from build123d import *

# Parameters (mm, degrees)
SKETCH_1_R                = 4
EXTRUDE_1_DEPTH           = 5
EXTRUDE_2_DEPTH           = 12
EXTRUDE_2_DEPTH_BACK      = 12
EXTRUDE_3_DEPTH           = 16
EXTRUDE_3_DEPTH_BACK      = 16
SKETCH_2_3_R              = 4
CUT_EXTRUDE_1_DEPTH       = 9
CUT_EXTRUDE_1_DEPTH_BACK  = 9
SKETCH_2_4_R              = 4
SKETCH_2_5_R              = 25
EXTRUDE_4_DEPTH           = 9
EXTRUDE_4_TAPER           = 30
EXTRUDE_4_OTHER_WAY_DEPTH = 9
EXTRUDE_4_OTHER_WAY_TAPER = 30


with BuildPart() as part:
    # Sketch 1 → Extrude 1 (new body)
    with BuildSketch(Plane.XY):
        with BuildLine():
            Line((21.5, -35), (-21.5, -35))
            ThreePointArc((-21.5, -35), (-24.328427125, -33.828427125), (-25.5, -31))
            Line((-25.5, -31), (-25.5, 31))
            ThreePointArc((-25.5, 31), (-24.328427125, 33.828427125), (-21.5, 35))
            Line((-21.5, 35), (21.5, 35))
            ThreePointArc((21.5, 35), (24.328427125, 33.828427125), (25.5, 31))
            Line((25.5, 31), (25.5, -31))
            ThreePointArc((25.5, -31), (24.328427125, -33.828427125), (21.5, -35))
        make_face()
        with Locations((-17.5, 26.5)):
            Circle(SKETCH_1_R, mode=Mode.SUBTRACT)
        with Locations((17.5, 26.5)):
            Circle(SKETCH_1_R, mode=Mode.SUBTRACT)
        with Locations((17.5, -26.5)):
            Circle(SKETCH_1_R, mode=Mode.SUBTRACT)
        with Locations((-17.5, -26.5)):
            Circle(SKETCH_1_R, mode=Mode.SUBTRACT)
    extrude(amount=EXTRUDE_1_DEPTH)

    # Sketch 2 → Extrude 2 (add, two sides: drawn at the far end of the back side and taken through both)
    with BuildSketch(Plane(origin=(0, 0, 0), x_dir=(0, 0, -1), z_dir=(1, 0, 0)).offset(-EXTRUDE_2_DEPTH_BACK)):
        with BuildLine():
            ThreePointArc((23.824417981, -16.040481733), (18, 0), (23.824417981, 16.040481733))
            Line((23.824417981, 16.040481733), (0, 31))
            Line((0, 31), (0, -31))
            Line((0, -31), (23.824417981, -16.040481733))
        make_face()
        with BuildLine():
            ThreePointArc((43, -4), (39, 0), (43, 4))
            Line((43, 4), (23.824417981, 16.040481733))
            ThreePointArc((23.824417981, 16.040481733), (18, 0), (23.824417981, -16.040481733))
            Line((23.824417981, -16.040481733), (43, -4))
        make_face()
    extrude(amount=EXTRUDE_2_DEPTH + EXTRUDE_2_DEPTH_BACK)

    # Sketch 2_3 → Extrude 3 (add, two sides: drawn at the far end of the back side and taken through both)
    with BuildSketch(Plane(origin=(0, 0, 0), x_dir=(0, 0, -1), z_dir=(1, 0, 0)).offset(-EXTRUDE_3_DEPTH_BACK)):
        with Locations((43, 0)):
            Circle(SKETCH_2_3_R)
    extrude(amount=EXTRUDE_3_DEPTH + EXTRUDE_3_DEPTH_BACK)

    # Sketch 2_4 → Cut-Extrude 1 (cut, two sides: drawn at the far end of the back side and taken through both)
    with BuildSketch(Plane(origin=(0, 0, 0), x_dir=(0, 0, -1), z_dir=(1, 0, 0)).offset(-CUT_EXTRUDE_1_DEPTH_BACK)):
        with BuildLine():
            ThreePointArc((23.824417981, -16.040481733), (18, 0), (23.824417981, 16.040481733))
            Line((23.824417981, 16.040481733), (0, 31))
            Line((0, 31), (0, -31))
            Line((0, -31), (23.824417981, -16.040481733))
        make_face()
        with BuildLine():
            ThreePointArc((43, -4), (39, 0), (43, 4))
            Line((43, 4), (23.824417981, 16.040481733))
            ThreePointArc((23.824417981, 16.040481733), (18, 0), (23.824417981, -16.040481733))
            Line((23.824417981, -16.040481733), (43, -4))
        make_face()
        with BuildLine():
            Line((23.824417981, 16.040481733), (43, 4))
            ThreePointArc((43, 4), (45.828427125, 2.828427125), (47, 0))
            ThreePointArc((47, 0), (45.828427125, -2.828427125), (43, -4))
            Line((43, -4), (23.824417981, -16.040481733))
            ThreePointArc((23.824417981, -16.040481733), (51.532597773, -23.498824976), (68, 0))
            ThreePointArc((68, 0), (51.532597773, 23.498824976), (23.824417981, 16.040481733))
        make_face()
        with Locations((43, 0)):
            Circle(SKETCH_2_4_R)
    extrude(amount=CUT_EXTRUDE_1_DEPTH + CUT_EXTRUDE_1_DEPTH_BACK, mode=Mode.SUBTRACT)

    # Sketch 2_5 → Extrude 4 (add)
    with BuildSketch(Plane(origin=(0, 0, 0), x_dir=(0, 0, -1), z_dir=(1, 0, 0))):
        with Locations((43, 0)):
            Circle(SKETCH_2_5_R)
    extrude(amount=EXTRUDE_4_DEPTH, taper=EXTRUDE_4_TAPER)

    # Sketch 2_5 → Extrude 4 other way (add)
    with BuildSketch(Plane(origin=(0, 0, 0), x_dir=(0, 0, -1), z_dir=(1, 0, 0))):
        with Locations((43, 0)):
            Circle(SKETCH_2_5_R)
    extrude(amount=-EXTRUDE_4_OTHER_WAY_DEPTH, taper=EXTRUDE_4_OTHER_WAY_TAPER)


solid = part.part
The listing builds one solid part. Answer for the finished solid, in the listing's coordinates (mm). A direction names the side the tool comes from. Coordinates: 2 decimals unless noted, no trailing zeros. Write each loop counter-clockwise with the first axis right and the second up, starting at its lowest first coordinate (ties: lowest second). Pieces come first, ordered by that corner, then holes. Notation, with made-up numbers: M 81,86.25 L 99,86.25 A28 cw 99,124.25 Z; hole C 12.5,63.5 d5. An arc over 180 degrees is marked long. Use one line per item in the form item = value.
Item 1: The mould has two halves that part along X. Classify faces 1 (the face through (0, 0, 5)), 2 (the face through (9, 0, -11)), 3 (the face through (-16, 0, -43)): released by +X, released by -X, zero draft, split by the parting line, or undercut.
Model answer:
face_1 = zero draft
face_2 = undercut
face_3 = released by -X
Item 2: Find the intervals of material crossed by probe 1 along Y at (x, z) = (-17.5, 2.3); probe 2 along X at (y, z) = (-26, 3); probe 3 along Z at (x, y) = (-6, -32), in increasing order.
Model answer:
probe_1 = -35 to -30.5, -22.5 to 22.5, 30.5 to 35
probe_2 = -25.5 to -21.47, -13.53 to 13.53, 21.47 to 25.5
probe_3 = 0 to 5
Item 3: Find section A-A, the plane x = 17.5. Give the vertices of the cut face in (y, z), plus the area to 3 significant figures.
Model answer:
outline = M -35,0 L -30.5,0 L -30.5,5 L -35,5 Z; M -22.5,0 L 22.5,0 L 22.5,5 L -22.5,5 Z; M 30.5,0 L 35,0 L 35,5 L 30.5,5 Z
area = 270 mm2
Item 4: Find section B-B, the plane y = -26.5. Give the vertices of the cut face in (x, z), plus the area to 3 significant figures.
Model answer:
outline = M -25.5,0 L -21.5,0 L -21.5,5 L -25.5,5 Z; M -13.5,0 L -12,0 L -12,-7.17 L -9,-7.17 L -9,0 L 9,0 L 9,-7.17 L 12,-7.17 L 12,0 L 13.5,0 L 13.5,5 L -13.5,5 Z; M 21.5,0 L 25.5,0 L 25.5,5 L 21.5,5 Z
area = 218 mm2
Item 5: For faces 4 (the face through (-9, 0, -49)), 5 (the face through (13.229, 1.201, -46.815)), 6 (the face through (-8.56, -12.2, -27.08)), 7 (the face through (-13.327, 1.201, -46.815)), determine the directions among +Z, -Z, +X, -X, +Y, -Y from which every point of the face is accessible in a straight line to the end or side of a thin tool.
Model answer:
face_4 = -Z, -X
face_5 = +X
face_6 = none
face_7 = -X
Item 6: Given P1, Ø5, axis at x = 7, y = -18.5, coming from the -Z side; P2, Ø6.5, axis at x = -17.5, y = 26.5, coming from the -Z side; P3, Ø2.5, axis at y = -0.5, z = -41.5, coming from the -X side; P4, Ø5, axis at x = -3, z = -45.5, coming from the -Y side, each flat-ended and moving along its own axis, determine where each tip first touches the part or whether it passes through.
Model answer:
P1 = -57.29
P2 = through
P3 = -16
P4 = -24.6
Item 7: Find section C-C, the plane z = -2. Give the vertices of the cut face in (x, y).
Model answer:
outline = M -12,-29.74 L -9,-29.74 L -9,29.74 L -12,29.74 Z; M 9,-29.74 L 12,-29.74 L 12,29.74 L 9,29.74 Z
Item 8: Find section D-D, the plane x = 3. Give the vertices of the cut face in (y, z).
Model answer:
outline = M -35,0 L 35,0 L 35,5 L -35,5 Z; C 0,-43 d46.54
